from build123d import *

# Parameters (mm, degrees)
SKETCH1_W                                      = 152.4
SKETCH1_H                                      = 127
BOSS_EXTRUDE1_DEPTH                            = 6.35
CUT_EXTRUDE1_DEPTH                             = 7.35
F_4_40_TAPPED_HOLE1_D                          = 2.2606
F_4_40_TAPPED_HOLE1_DEPTH                      = 7.5946
F_4_40_TAPPED_HOLE1_TIP                        = 0.679152758
CBORE_FOR_4_SOCKET_HEAD_CAP_SCREW1_D           = 3.2639
CBORE_FOR_4_SOCKET_HEAD_CAP_SCREW1_DEPTH       = 7.5946
CBORE_FOR_4_SOCKET_HEAD_CAP_SCREW1_CBORE_D     = 5.55752
CBORE_FOR_4_SOCKET_HEAD_CAP_SCREW1_CBORE_DEPTH = 2.8448
CBORE_FOR_4_SOCKET_HEAD_CAP_SCREW1_TIP         = 0.980574487
CBORE_FOR_4_SOCKET_HEAD_CAP_SCREW2_D           = 3.2639
CBORE_FOR_4_SOCKET_HEAD_CAP_SCREW2_DEPTH       = 7.5946
CBORE_FOR_4_SOCKET_HEAD_CAP_SCREW2_CBORE_D     = 5.55752
CBORE_FOR_4_SOCKET_HEAD_CAP_SCREW2_CBORE_DEPTH = 2.8448
CBORE_FOR_4_SOCKET_HEAD_CAP_SCREW2_TIP         = 0.980574487
F_4_40_TAPPED_HOLE2_D                          = 2.2606
F_4_40_TAPPED_HOLE2_DEPTH                      = 7.5946
F_4_40_TAPPED_HOLE2_TIP                        = 0.679152758
FILLET1_R                                      = 3.175


with BuildPart() as part:
    # Sketch1 → Boss-Extrude1 (new body)
    with BuildSketch(Plane.XY):
        Rectangle(SKETCH1_W, SKETCH1_H)
    extrude(amount=BOSS_EXTRUDE1_DEPTH)

    # Sketch2 → Cut-Extrude1 (cut, through all)
    with BuildSketch(Plane.XY.offset(6.35)):
        Polygon((63.5, 50.8), (63.5, -50.8), (12.7, 1.254738493), align=None)
        Polygon((-63.5, -50.8), (-12.7, 1.254738493), (-63.5, 50.8), align=None)
        Polygon((38.1, -50.8), (-38.1, -50.8), (0, -11.758946131), align=None)
        Polygon((-38.1, 50.8), (0, 11.758946131), (38.1, 50.8), align=None)
    extrude(amount=-CUT_EXTRUDE1_DEPTH, mode=Mode.SUBTRACT)

    # #4-40 Tapped Hole1
    with Locations(Plane(origin=(0, -63.5, 0), x_dir=(-1, 0, 0), z_dir=(0, -1, 0))):
        with Locations((-73.025, -3.175), (73.025, -3.175)):
            Hole(F_4_40_TAPPED_HOLE1_D / 2, depth=F_4_40_TAPPED_HOLE1_DEPTH)
            with Locations((0, 0, -(F_4_40_TAPPED_HOLE1_DEPTH + F_4_40_TAPPED_HOLE1_TIP / 2))):  # 118° drill point
                Cone(0, F_4_40_TAPPED_HOLE1_D / 2, F_4_40_TAPPED_HOLE1_TIP, mode=Mode.SUBTRACT)

    # CBORE for #4 Socket Head Cap Screw1
    with Locations(Plane(origin=(0, 0, 0), x_dir=(-1, 0, 0), z_dir=(0, 0, -1))):
        with Locations((73.025, 0), (73.025, 50.8), (-73.025, 50.8), (-73.025, 0), (-73.025, -50.8), (73.025, -50.8)):
            CounterBoreHole(CBORE_FOR_4_SOCKET_HEAD_CAP_SCREW1_D / 2, CBORE_FOR_4_SOCKET_HEAD_CAP_SCREW1_CBORE_D / 2, CBORE_FOR_4_SOCKET_HEAD_CAP_SCREW1_CBORE_DEPTH, depth=CBORE_FOR_4_SOCKET_HEAD_CAP_SCREW1_DEPTH)
            with Locations((0, 0, -(CBORE_FOR_4_SOCKET_HEAD_CAP_SCREW1_DEPTH + CBORE_FOR_4_SOCKET_HEAD_CAP_SCREW1_TIP / 2))):  # 118° drill point
                Cone(0, CBORE_FOR_4_SOCKET_HEAD_CAP_SCREW1_D / 2, CBORE_FOR_4_SOCKET_HEAD_CAP_SCREW1_TIP, mode=Mode.SUBTRACT)

    # CBORE for #4 Socket Head Cap Screw2
    with Locations(Plane(origin=(0, 0, 0), x_dir=(-1, 0, 0), z_dir=(0, 0, -1))):
        with Locations((0, 0)):
            CounterBoreHole(CBORE_FOR_4_SOCKET_HEAD_CAP_SCREW2_D / 2, CBORE_FOR_4_SOCKET_HEAD_CAP_SCREW2_CBORE_D / 2, CBORE_FOR_4_SOCKET_HEAD_CAP_SCREW2_CBORE_DEPTH, depth=CBORE_FOR_4_SOCKET_HEAD_CAP_SCREW2_DEPTH)
            with Locations((0, 0, -(CBORE_FOR_4_SOCKET_HEAD_CAP_SCREW2_DEPTH + CBORE_FOR_4_SOCKET_HEAD_CAP_SCREW2_TIP / 2))):  # 118° drill point
                Cone(0, CBORE_FOR_4_SOCKET_HEAD_CAP_SCREW2_D / 2, CBORE_FOR_4_SOCKET_HEAD_CAP_SCREW2_TIP, mode=Mode.SUBTRACT)

    # #4-40 Tapped Hole2
    with Locations(Plane(origin=(0, 63.5, 0), x_dir=(1, 0, 0), z_dir=(0, 1, 0))):
        with Locations((-73.025, -3.175), (73.025, -3.175)):
            Hole(F_4_40_TAPPED_HOLE2_D / 2, depth=F_4_40_TAPPED_HOLE2_DEPTH)
            with Locations((0, 0, -(F_4_40_TAPPED_HOLE2_DEPTH + F_4_40_TAPPED_HOLE2_TIP / 2))):  # 118° drill point
                Cone(0, F_4_40_TAPPED_HOLE2_D / 2, F_4_40_TAPPED_HOLE2_TIP, mode=Mode.SUBTRACT)

    # Fillet1
    fillet1_edges = [part.edges().sort_by_distance(p)[0] for p in [
        (0, -11.758946131, 3.175),
        (38.1, -50.8, 3.175),
        (-38.1, -50.8, 3.175),
        (-63.5, -50.8, 3.175),
        (-63.5, 50.8, 3.175),
        (-12.7, 1.254738493, 3.175),
        (-38.1, 50.8, 3.175),
        (38.1, 50.8, 3.175),
        (0, 11.758946131, 3.175),
        (12.7, 1.254738493, 3.175),
        (63.5, 50.8, 3.175),
        (63.5, -50.8, 3.175),
    ]]
    fillet(fillet1_edges, radius=FILLET1_R)


solid = part.part
Build history of the part. All positions in model axes, mm. A direction names the side the tool comes from. Give positions to 0.01 mm unless a question says otherwise; leave off trailing zeros. Write each loop counter-clockwise with the first axis right and the second up, starting at its lowest first coordinate (ties: lowest second). Pieces come first, ordered by that corner, then holes. Notation, with made-up numbers: (-27.5, -12.5) - (21.5, -12.5) arc R19 ccw to (21.5, 4.5) - close; hole circle Ø5 at (59, 64.5). An arc over 180 degrees is marked (long way). Use one line per item in the form item = value. Start each with the question number.
1. Two-plate mould, pull along X, no slides. Class faces 3 (the face through (63.5, 1, 3)), 4 (the face through (-1, -13, 0)): released by +X, released by -X, zero draft, split by the parting line, or undercut.
2. Drop flat-ended pins along their axis: pin 1 Ø2 at (x, y) = (0, 0) entering from -Z; pin 2 Ø1.7 at (x, y) = (-72, 0) entering from -Z. Give the stop position or say it passes through.
3. 3-axis set-ups, long thin cutter, end or side, ignore diameter. For faces 1 (the face through (-70.25, 0.12, 1.4)), 2 (the face through (36.79, -23.43, 3.22)): which of +Z, -Z, +X, -X, +Y, -Y reach the whole face in a straight line?
4. Band-saw the part on D-D on x = -60. Write the cut outline in (y, z).
5. Band-saw the part on C-C on z = 1. Count the separate pieces of the cut face and the enclosed holes in it, plus the area to 3 significant figures.
6. Band-saw the part on A-A on x = 0. Write the cut outline in (y, z).
7. Probe line 1 (Y direction, x = 33, z = 1.75); line 2 (X direction, y = -17, z = 1.5); line 3 (Y direction, x = 3.5, z = 0.75). List the from-to ranges inside material, lowest first. Write a range as [from, to].
8. Band-saw the part on B-B on y = -17.5. Write the cut outline in (x, z).
Conclusion:
q1.face_3 = undercut
q1.face_4 = zero draft
q2.pin_1 = through
q2.pin_2 = 2.84
q3.face_1 = -Z
q3.face_2 = +Z, -Z
q4.outline = (-63.5, 0) - (-46.16, 0) - (-46.16, 6.35) - (-63.5, 6.35) - close; (46.43, 0) - (63.5, 0) - (63.5, 6.35) - (46.43, 6.35) - close
q5.separate_pieces = 1
q5.enclosed_holes = 11
q5.area = 11,200 mm²
q6.outline = (-63.5, 0) - (-50.8, 0) - (-50.8, 6.35) - (-63.5, 6.35) - close; (-13.13, 0) - (-2.78, 0) - (-2.78, 2.84) - (-1.63, 2.84) - (-1.63, 6.35) - (-13.13, 6.35) - close; (1.63, 2.84) - (2.78, 2.84) - (2.78, 0) - (13.13, 0) - (13.13, 6.35) - (1.63, 6.35) - close; (50.8, 0) - (63.5, 0) - (63.5, 6.35) - (50.8, 6.35) - close
q7.line_1 = [-63.5, -49.66], [-45.59, -19.55], [21.05, 45.59], [49.66, 63.5]
q7.line_2 = [-76.2, -63.5], [-30.51, -5.11], [5.11, 30.51], [63.5, 76.2]
q7.line_3 = [-63.5, -50.8], [-15.35, 15.35], [50.8, 63.5]
q8.outline = (-76.2, 0) - (-63.5, 0) - (-63.5, 6.35) - (-76.2, 6.35) - close; (-31, 0) - (-5.6, 0) - (-5.6, 6.35) - (-31, 6.35) - close; (5.6, 0) - (31, 0) - (31, 6.35) - (5.6, 6.35) - close; (63.5, 0) - (76.2, 0) - (76.2, 6.35) - (63.5, 6.35) - close
